from build123d import *

# Parameters (mm, degrees)
F0_R          = 50
F0_R_2        = 7.5
F0_R_3        = 4.125
F1_DEPTH      = 30
F3_DEPTH      = 12
F4_R          = 2
F5_DEPTH      = 25
F5_DEPTH_BACK = 25
F8_R          = 16
F9_DEPTH      = 44.4
F10_R         = 60
F10_R_2       = 4
F10_R_3       = 50
F11_DEPTH     = 3
F13_START     = -18.6
F12_R         = 2
F13_DEPTH     = 76


with BuildPart() as f1:
    # F0 (on Top) → F1 (new body)
    with BuildSketch(Plane.XY):
        Circle(F0_R)
        with BuildLine():
            ThreePointArc((-29.5606389839, -23.0992315385), (-36.6970313958, -21.1870409548), (-34.7848408122, -14.050648543))
            ThreePointArc((-34.7848408122, -14.050648543), (-34.4741747133, -13.884984547), (-34.1530557988, -13.7406217149))
            Line((-34.1530557988, -13.7406217149), (-11.8039810165, -2.7735797331))
            ThreePointArc((-11.8039810165, -2.7735797331), (-8.3039810165, -2.7735797331), (-6.5539810165, -5.8046686463))
            ThreePointArc((-6.5539810165, -5.8046686463), (-7.0228921033, -7.5546686463), (-8.3039810165, -8.8357575596))
            Line((-8.3039810165, -8.8357575596), (-28.9762553683, -22.7071030812))
            ThreePointArc((-28.9762553683, -22.7071030812), (-29.2618367055, -22.9130188027), (-29.5606389839, -23.0992315385))
        make_face(mode=Mode.SUBTRACT)
        with BuildLine():
            ThreePointArc((34.7848408122, -14.050648543), (36.6970313958, -15.9628391266), (37.3969417263, -18.5749400407))
            ThreePointArc((37.3969417263, -18.5749400407), (34.7848408122, -23.0992315385), (29.5606389839, -23.0992315385))
            ThreePointArc((29.5606389839, -23.0992315385), (29.2618367055, -22.9130188027), (28.9762553683, -22.7071030812))
            Line((28.9762553683, -22.7071030812), (8.3039810165, -8.8357575596))
            ThreePointArc((8.3039810165, -8.8357575596), (7.0228921033, -4.0546686463), (11.8039810165, -2.7735797331))
            Line((11.8039810165, -2.7735797331), (34.1530557988, -13.7406217149))
            ThreePointArc((34.1530557988, -13.7406217149), (34.4741747133, -13.884984547), (34.7848408122, -14.050648543))
        make_face(mode=Mode.SUBTRACT)
        Circle(F0_R_2, mode=Mode.SUBTRACT)
        with BuildLine():
            ThreePointArc((-5.2242018282, 37.1498800814), (0, 42.3740819097), (5.2242018282, 37.1498800814))
            ThreePointArc((5.2242018282, 37.1498800814), (5.2123380078, 36.7980033497), (5.1768004305, 36.4477247961))
            Line((5.1768004305, 36.4477247961), (3.5, 11.6093372926))
            ThreePointArc((3.5, 11.6093372926), (0, 8.1093372926), (-3.5, 11.6093372926))
            Line((-3.5, 11.6093372926), (-5.1768004305, 36.4477247961))
            ThreePointArc((-5.1768004305, 36.4477247961), (-5.2123380078, 36.7980033497), (-5.2242018282, 37.1498800814))
        make_face(mode=Mode.SUBTRACT)
        Circle(F0_R_2)
        Circle(F0_R_3, mode=Mode.SUBTRACT)
    extrude(amount=F1_DEPTH)

    # F0 (on Top) → F3 (join)
    with BuildSketch(Plane.XY):
        Circle(F0_R_2)
        Circle(F0_R_3, mode=Mode.SUBTRACT)
    extrude(amount=-F3_DEPTH)

    # F4 (on Right) → F5 (cut, two sides)
    with BuildSketch(Plane.YZ) as f5_sk:
        with Locations((0, -8)):
            Circle(F4_R)
    extrude(amount=F5_DEPTH, mode=Mode.SUBTRACT)
    extrude(f5_sk.sketch, amount=-F5_DEPTH_BACK, mode=Mode.SUBTRACT)

    # F6 (on Right) → F7 (revolve, cut)
    with BuildSketch(Plane.YZ):
        with BuildLine():
            Line((53.9439544082, 27), (50, 27))
            ThreePointArc((50, 27), (45.7573593129, 25.2426406871), (44, 21))
            Line((44, 21), (44, 9))
            ThreePointArc((44, 9), (45.7573593129, 4.7573593129), (50, 3))
            Line((50, 3), (53.9439544082, 3))
            Line((53.9439544082, 3), (53.9439544082, 27))
        make_face()
    revolve(axis=Axis((0, 0, 17.027027905), (0, 0, 1)), mode=Mode.SUBTRACT)

    # F8 (on face) → F9 (cut)
    with BuildSketch(Plane.XY.offset(30)):
        with Locations((-22.635814867, 13.0687938068)):
            Circle(F8_R)
        with Locations((22.635814867, 13.0687938068)):
            Circle(F8_R)
        with Locations((0, -26.1375876136)):
            Circle(F8_R)
    extrude(amount=-F9_DEPTH, mode=Mode.SUBTRACT)

    # F10 (on face) → F11 (join)
    with BuildSketch(Plane.XY.offset(30)):
        Circle(F10_R)
        with Locations((-32.0342962499, -44.0914261934)):
            Circle(F10_R_2, mode=Mode.SUBTRACT)
        with Locations((-51.8325801381, -16.8414261934)):
            Circle(F10_R_2, mode=Mode.SUBTRACT)
        with Locations((0, -54.5)):
            Circle(F10_R_2, mode=Mode.SUBTRACT)
        with Locations((32.0342962499, -44.0914261934)):
            Circle(F10_R_2, mode=Mode.SUBTRACT)
        with Locations((51.8325801381, -16.8414261934)):
            Circle(F10_R_2, mode=Mode.SUBTRACT)
        with Locations((-51.8325801381, 16.8414261934)):
            Circle(F10_R_2, mode=Mode.SUBTRACT)
        with Locations((-32.0342962499, 44.0914261934)):
            Circle(F10_R_2, mode=Mode.SUBTRACT)
        Circle(F10_R_3, mode=Mode.SUBTRACT)
        with Locations((51.8325801381, 16.8414261934)):
            Circle(F10_R_2, mode=Mode.SUBTRACT)
        with Locations((0, 54.5)):
            Circle(F10_R_2, mode=Mode.SUBTRACT)
        with Locations((32.0342962499, 44.0914261934)):
            Circle(F10_R_2, mode=Mode.SUBTRACT)
    extrude(amount=-F11_DEPTH)

    # F12 (on Front) → F13 (cut)
    with BuildSketch(Plane.XZ.offset(F13_START)):
        with Locations((0, 23.7334519625)):
            Circle(F12_R)
    extrude(amount=-F13_DEPTH, mode=Mode.SUBTRACT)


solid = f1.part
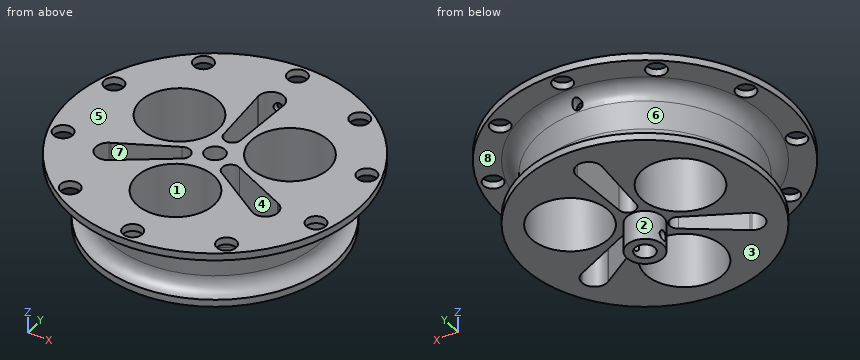
Work out the finished part from the listing and answer in its coordinate system (mm). Face numbers are marked on the shaded views. A direction names the side the tool comes from. Round coordinates to 2 decimals unless told otherwise and drop trailing zeros. Write each loop counter-clockwise with the first axis right and the second up, starting at its lowest first coordinate (ties: lowest second). Pieces come first, ordered by that corner, then holes.
1) A cutting plane is placed at C-C (x = 0). Give the number of separate pieces and of enclosed holes in the cut face, plus the area to 3 significant figures.
2) A cutting plane is placed at D-D (z = 10.5). Give the vertices of the cut face in (x, y) (3 decimals).
3) A tool of negligible diameter and unlimited length cuts with its end or side. For the marked faces 5, 6, 7 and 8, from which of +Z, -Z, +X, -X, +Y, -Y can it reach the whole face along a straight path? Write none if from no direction.
4) Straight lines are drawn through the part: line 1 (Y direction, x = 0, z = 15.25) (3 decimals); line 2 (Z direction, x = 0, y = 43); line 3 (Y direction, x = -22, z = 22). For each, find the intervals that lie inside material, in ascending order.
5) A cutting plane is placed at B-B (y = -54.5). Give the vertices of the cut face in (x, z), plus the area to 3 significant figures.
6) A cutting plane is placed at A-A (z = -8). Give the vertices of the cut face in (x, y) (3 decimals).
7) Given pin 1 Ø3 at (x, z) = (-8.5, 11) entering from +Y; pin 2 Ø1.5 at (y, z) = (-23, -0.5) entering from -X; pin 3 Ø5 at (y, z) = (0, -8) entering from +X; pin 4 Ø6.5 at (x, y) = (0, 54.5) entering from -Z, each flat-ended and moving along its own axis, determine where each tip first touches the part or whether it passes through.
8) The mould has two halves that part along X. Classify the marked faces 1, 2, 3 and 4: pulls with the +X half, pulls with the -X half, needs draft (parallel to the pull), parting line crosses it, or undercut.
Completed:
1. separate pieces: 7
1. enclosed holes: 0
1. area: 591 mm2
2. outline: circle Ø88 at (0, 0); hole circle Ø32 at (-22.636, 13.069); hole (-34.153, -13.741) arc R5.224 ccw (long way) to (-28.976, -22.707) - (-8.304, -8.836) arc R3.5 ccw to (-11.804, -2.774) - close; hole circle Ø32 at (0, -26.138); hole (-5.177, 36.448) - (-3.5, 11.609) arc R3.5 ccw to (3.5, 11.609) - (5.177, 36.448) arc R5.224 ccw (long way) to start; hole circle Ø8.25 at (0, 0); hole circle Ø32 at (22.636, 13.069); hole (8.304, -8.836) - (28.976, -22.707) arc R5.224 ccw (long way) to (34.153, -13.741) - (11.804, -2.774) arc R3.5 ccw to start
3. face 5: +Z, +X, -X, +Y, -Y
3. face 6: none
3. face 7: +Z, -Z
3. face 8: -Z
4. line 1: y = -44 to -42.138, -10.138 to -4.125, 4.125 to 8.109, 42.374 to 44
4. line 2: z = 0 to 21.73, 25.73 to 30
4. line 3: y = -38.2 to -18.03, -7.78 to -2.92, 29.06 to 38.2
5. outline: (-25.09, 27) - (-4, 27) - (-4, 30) - (-25.09, 30) - close; (4, 27) - (25.09, 27) - (25.09, 30) - (4, 30) - close
5. area: 127 mm2
6. outline: (-7.228, -2) arc R7.5 ccw to (7.228, -2) - (3.608, -2) arc R4.125 cw to (-3.608, -2) - close; (-7.228, 2) - (-3.608, 2) arc R4.125 cw to (3.608, 2) - (7.228, 2) arc R7.5 ccw to start
7. pin 1: stops at y = 43.44
7. pin 2: stops at x = -44.68
7. pin 3: stops at x = 7.5
7. pin 4: passes through
8. face 1: undercut
8. face 2: parting line crosses it
8. face 3: needs draft
8. face 4: undercut
